```python
from build123d import *

# Parameters (mm, degrees)
F1_DEPTH = 35
F2_R     = 7.5
F3_DEPTH = 0.6
F4_R     = 2
F5_R     = 5
F6_DEPTH = 25.001


with BuildPart() as f1:
    # F0 (on Front) → F1 (new body)
    with BuildSketch(Plane.XZ):
        Polygon((-12.5, 0), (0, 0), (12.5, 0), (12.5, 20), (11.5, 20), (11.5, 1), (0, 1), (-11.5, 1), (-11.5, 20), (-12.5, 20), align=None)
    extrude(amount=F1_DEPTH)

    # F2 (on face) → F3 (cut)
    with BuildSketch(Plane.XY.offset(1)):
        with Locations((0, -8.5)):
            Circle(F2_R)
        with Locations((0, -26.5)):
            Circle(F2_R)
    extrude(amount=-F3_DEPTH, mode=Mode.SUBTRACT)

    # F4
    f4_edges = [f1.edges().sort_by_distance(p)[0] for p in [
        (-11.5, -17.5, 1),
        (11.5, -17.5, 1),
        (-12, -35, 20),
        (12, -35, 20),
        (12, 0, 20),
        (-12, 0, 20),
    ]]
    fillet(f4_edges, radius=F4_R)

    # F5 (on face) → F6 (cut, through all)
    with BuildSketch(Plane(origin=(-12.5, 0, 0), x_dir=(0, -1, 0), z_dir=(-1, 0, 0))):
        with Locations((17.5, 9)):
            Circle(F5_R)
    extrude(amount=-F6_DEPTH, mode=Mode.SUBTRACT)


solid = f1.part
```
Verification items for the finished model (mm, model axes). A direction names the side the tool comes from. Coordinates: 2 decimals unless noted, no trailing zeros. Order: outer loops, then holes, each group sorted by start corner. A loop starts at its lowest first (then second) coordinate and runs counter-clockwise, first axis right, second up. Notation, with made-up numbers: (40.5, 76.25) - (62.5, 76.25) arc R27 cw to (62.5, 99.25) - close; hole circle Ø11 at (-38.5, 55). An arc over 180 degrees is marked (long way). Return JSON: item names as keys, results as strings.
(1) Section check D-D, the plane x = 2. Record the cut outline in (y, z), and give its area (3 significant figures).
Filled sheet:
{"outline": "(-35, 0) - (0, 0) - (0, 1) - (-1.27, 1) - (-1.27, 0.4) - (-15.73, 0.4) - (-15.73, 1) - (-19.27, 1) - (-19.27, 0.4) - (-33.73, 0.4) - (-33.73, 1) - (-35, 1) - close", "area": "17.7 mm^2"}
(2) Go/stop test with flat-tipped pins: pin 1 (7.5 mm diameter, centred on x = 3, y = -6, fed in from +Z); pin 2 (9 mm diameter, centred on y = -17.5, z = 9, fed in from -X); pin 3 (2 mm diameter, centred on x = -2.5, y = -8.5, fed in from +Z). Record where each tip stops, or that it passes through.
Filled sheet:
{"pin 1": "stops at z = 1", "pin 2": "passes through", "pin 3": "stops at z = 0.4"}
(3) Access from +Z, -Z, +X, -X, +Y, -Y to the whole of each face (thin tool, end or side, straight path). Record for faces 1 (the flat face through (11.5, -17, 15)), 2 (the cylindrical face through (-12.007, -16.849, 13.957)), 3 (the flat face through (0, -8, 0.4)).
Filled sheet:
{"face 1": "+Z, +Y, -Y", "face 2": "+X, -X", "face 3": "+Z"}
(4) Section check C-C, the plane y = -26.5. Record the cut outline in (x, z), and give its area (3 significant figures).
Filled sheet:
{"outline": "(-12.5, 0) - (12.5, 0) - (12.5, 20) - (11.5, 20) - (11.5, 3) arc R2 cw to (9.5, 1) - (7.5, 1) - (7.5, 0.4) - (-7.5, 0.4) - (-7.5, 1) - (-9.5, 1) arc R2 cw to (-11.5, 3) - (-11.5, 20) - (-12.5, 20) - close", "area": "55.7 mm^2"}
(5) Mould release check, pull along Z, two halves, no side actions. Record for faces 4 (the cylindrical face through (-0.976, -19.064, 0.704)), 5 (the flat face through (-12, -17, 20)), 6 (the cylindrical face through (11.993, -16.849, 13.957)): pulls with the +Z half, pulls with the -Z half, needs draft (parallel to the pull), parting line crosses it, or undercut.
Filled sheet:
{"face 4": "needs draft", "face 5": "pulls with the +Z half", "face 6": "undercut"}
(6) Section check A-A, the plane y = -17.5. Record the cut outline in (x, z), and give its area (3 significant figures).
Filled sheet:
{"outline": "(-12.5, 0) - (12.5, 0) - (12.5, 4) - (11.5, 4) - (11.5, 3) arc R2 cw to (9.5, 1) - (-9.5, 1) arc R2 cw to (-11.5, 3) - (-11.5, 4) - (-12.5, 4) - close; (-12.5, 14) - (-11.5, 14) - (-11.5, 20) - (-12.5, 20) - close; (11.5, 14) - (12.5, 14) - (12.5, 20) - (11.5, 20) - close", "area": "44.7 mm^2"}
(7) Thickness scan on line 1 along Y through (x, z) = (0, 0.85); line 2 along Z through (x, y) = (12.25, -17.5); line 3 along X through (y, z) = (-15.5, 17.5). Record the ranges inside material, lowest first.
Filled sheet:
{"line 1": "y = -35 to -34, -19 to -16, -1 to 0", "line 2": "z = 0 to 4, 14 to 20", "line 3": "x = -12.5 to -11.5, 11.5 to 12.5"}
(8) Section check B-B, the plane z = 9. Record the cut outline in (x, y).
Filled sheet:
{"outline": "(-12.5, -35) - (-11.5, -35) - (-11.5, -22.5) - (-12.5, -22.5) - close; (-12.5, -12.5) - (-11.5, -12.5) - (-11.5, 0) - (-12.5, 0) - close; (11.5, -35) - (12.5, -35) - (12.5, -22.5) - (11.5, -22.5) - close; (11.5, -12.5) - (12.5, -12.5) - (12.5, 0) - (11.5, 0) - close"}
